from build123d import *

# Parameters (mm, degrees)
F0_R     = 3
F1_DEPTH = 1
F2_R     = 2.5
F3_DEPTH = 6
F4_R     = 2.5
F5_W     = 1.9698908329
F5_H     = 6.6161441393
F5_W_2   = 2.2700465526
F6_DEPTH = 12.5
F7_R     = 1
F8_DEPTH = 4.001


with BuildPart() as f1:
    # F0 (on Top) → F1 (new body)
    with BuildSketch(Plane.XY):
        Circle(F0_R)
    extrude(amount=F1_DEPTH)

    # F2 (on face) → F3 (join)
    with BuildSketch(Plane.XY.offset(1)):
        Circle(F2_R)
    extrude(amount=F3_DEPTH)

    # F4
    f4_edges = [f1.edges().sort_by_distance(p)[0] for p in [
        (-2.5, 0, 7),
    ]]
    fillet(f4_edges, radius=F4_R)

    # F5 (on Front) → F6 (cut, symmetric)
    with BuildSketch(Plane.XZ):
        with Locations((-1.9849454165, 4.3080720697)):
            Rectangle(F5_W, F5_H)
        with Locations((2.1350232763, 4.3080720697)):
            Rectangle(F5_W_2, F5_H)
    extrude(amount=F6_DEPTH, both=True, mode=Mode.SUBTRACT)

    # F7 (on face) → F8 (cut, through all)
    with BuildSketch(Plane(origin=(-1, 0, 0), x_dir=(0, -1, 0), z_dir=(-1, 0, 0))):
        with Locations((0, 4.5)):
            Circle(F7_R)
    extrude(amount=-F8_DEPTH, mode=Mode.SUBTRACT)


solid = f1.part
Can you work these out from the model? Positions are in its coordinate system, mm. A direction names the side the tool comes from. Give positions to 0.01 mm unless a question says otherwise; leave off trailing zeros. Loops run counter-clockwise (first coordinate to the right, second up) from the corner with the lowest first, then second, coordinate; pieces in that order, holes last. Notation, with made-up numbers: (52.25, -38.5) - (73.25, -38.5) arc R15 ccw to (73.25, -15.5) - close; hole circle Ø5 at (78.25, 30). An arc over 180 degrees is marked (long way). Return JSON: item names as keys, results as strings.
1. We'd pull the mould along Y, two halves only. Please class faces 1 (the face through (-3, 0.1, 0.5)), 2 (the face through (-0.01, 0.13, 5.49)), 3 (the face through (0, -2.5, 2.7)), 4 (the face through (0, 0, 0)): +Y half, -Y half, draft (parallel to the pull), parting line (faces both ways), or undercut.
Output values:
{"face 1": "parting line", "face 2": "undercut", "face 3": "-Y half", "face 4": "draft"}
2. I want a section at A-A on y = 0. Please give me the cut outline in (x, z).
Output values:
{"outline": "(-3, 0) - (3, 0) - (3, 1) - (1, 1) - (1, 3.5) - (-1, 3.5) - (-1, 1) - (-3, 1) - close; (-1, 5.5) - (1, 5.5) - (1, 6.79) arc R2.5 ccw to (-1, 6.79) - close"}
3. I want a section at D-D on y = 1.15. Please give me the cut outline in (x, z).
Output values:
{"outline": "(-2.77, 0) - (2.77, 0) - (2.77, 1) - (1, 1) - (1, 6.48) arc R2.22 ccw to (-1, 6.48) - (-1, 1) - (-2.77, 1) - close"}
4. I want a section at B-B on z = 5.25. Please give me the cut outline in (x, y), and give its area (3 significant figures).
Output values:
{"outline": "(-1, -2.17) arc R2.38 ccw to (1, -2.17) - (1, -0.66) - (-1, -0.66) - close; (-1, 0.66) - (1, 0.66) - (1, 2.17) arc R2.38 ccw to (-1, 2.17) - close", "area": "6.61 mm²"}
5. I'm going to push flat-ended pins straight in: pin 1 Ø3.5 at (y, z) = (0, 4.5) entering from +X; pin 2 Ø2 at (y, z) = (-1, 4.5) entering from -X. Where does each tip first touch, or does it pass through?
Output values:
{"pin 1": "stops at x = 1", "pin 2": "stops at x = -1"}
6. If I drill on line 1 (Z direction, x = -0.1, y = 0); line 2 (X direction, y = 0.7, z = 6.25); line 3 (Z direction, x = 1.8, y = 1.7), over which ranges is the centre line in solid material (lowest first)?
Output values:
{"line 1": "z = 0 to 3.5, 5.5 to 7", "line 2": "x = -1 to 1", "line 3": "z = 0 to 1"}
7. I want a section at C-C on x = 0. Please give me the cut outline in (y, z), and give its area (3 significant figures).
Output values:
{"outline": "(-3, 0) - (3, 0) - (3, 1) - (2.5, 1) - (2.5, 4.5) arc R2.5 ccw to (-2.5, 4.5) - (-2.5, 1) - (-3, 1) - close; hole circle Ø2 at (0, 4.5)", "area": "30.2 mm²"}
8. For faces 5 (the face through (-1, 0, 3)), 6 (the face through (1, 0, 3)), 7 (the face through (0, 2.5, 2.7)), which set-ups out of +Z, -Z, +X, -X, +Y, -Y let a thin tool reach every point of the face, with its end or its side?
Output values:
{"face 5": "+Z, -X, +Y, -Y", "face 6": "+Z, +X, +Y, -Y", "face 7": "+Z, +Y"}
